Design review of the part built by this model. Coordinates are the model's own, in mm. A direction names the side the tool comes from. Round coordinates to 2 decimals unless told otherwise and drop trailing zeros. Loops run counter-clockwise (first coordinate to the right, second up) from the corner with the lowest first, then second, coordinate; pieces in that order, holes last. Notation, with made-up numbers: (83.5, 47.5) - (96.5, 47.5) arc R32 cw to (96.5, 86.5) - close; hole circle Ø5 at (33.5, 43). An arc over 180 degrees is marked (long way). Use one line per item in the form item = value. Start each with the question number.
(1) We need section B-B, the plane x = 23. Write out the cut boundary in (y, z).
(2) We need section D-D, the plane z = -26. Write out the cut boundary in (x, y).
(3) We need section C-C, the plane y = 10.5. Write out the cut boundary in (x, z), then the cut area to 3 significant figures.
(4) The part is to be moulded in two halves that separate along X. For faces 5 (the cylindrical face through (5.28, 5.92, 15.98)), 6 (the flat face through (45.311, 7, -40)), 7 (the flat face through (19, 2, -60.058)), say which applies: released by +X, released by -X, zero draft, split by the parting line, or undercut.
(5) Wall thickness on probe 1 along Z at (x, y) = (27.5, 1.75); probe 2 along X at (y, z) = (9.25, 15); probe 3 along X at (y, z) = (2, -98): over which ranges is each line inside the solid? List them lowest first. Write a range as [from, to].
(6) For pin 1 (3 mm diameter, centred on x = 7, z = 0, fed in from +Y); pin 2 (1 mm diameter, centred on x = 9.5, y = 13, fed in from +Z), all flat-tipped, find the tip position at first contact; note any pin that passes through.
(7) Machinability: for faces 1 (the flat face through (19, 12, 4)), 2 (the flat face through (19, 4, -41)), 3 (the flat face through (18, 14, -41)), 4 (the flat face through (19, 12, -85)), which of the approach directions +Z, -Z, +X, -X, +Y, -Y give a long, thin tool a straight path to every point of the face, cutting with its end or side? Answer none if there is none.
(8) We need section A-A, the plane y = 1.5. Write out the cut boundary in (x, z), then the cut area to 3 significant figures.
Autodesk Inventor part; units mm, degrees
ref_plane "YZ Plane" through (0, 0, 0) normal (1, 0, 0) x (0, 1, 0)
ref_plane "XZ Plane" through (0, 0, 0) normal (0, 1, 0) x (-1, 0, 0)
ref_plane "XY Plane" through (0, 0, 0) normal (0, 0, 1) x (1, 0, 0)
sketch "Sketch1" plane through (0, 0, 0) normal (0, 1, 0) x (-1, 0, 0)
  line L0 (3.6894, 22.9423) -> (-40.3106, 22.9423)
  line L1 (-45.3106, 17.9423) -> (-45.3106, -100.0577)
  line L2 (-40.3106, -105.0577) -> (3.6894, -105.0577)
  line L3 (8.6894, -100.0577) -> (8.6894, 17.9423)
  arc A0 (8.6894, 17.9423) -> (3.6894, 22.9423) centre (3.6894, 17.9423) ccw
  arc A1 (3.6894, -105.0577) -> (8.6894, -100.0577) centre (3.6894, -100.0577) ccw
  arc A2 (-40.3106, 22.9423) -> (-45.3106, 17.9423) centre (-40.3106, 17.9423) ccw
  arc A3 (-45.3106, -100.0577) -> (-40.3106, -105.0577) centre (-40.3106, -100.0577) ccw
  circle A4 centre (-1.3106, 12.9423) radius 5
  circle A5 centre (-1.3106, -95.0577) radius 5
  circle A6 centre (-35.3106, 12.9423) radius 5
  circle A7 centre (-35.3106, -95.0577) radius 5
  point P0 (0, 0)
  point P1 (-45.3106, -105.0577)
  point P2 (-45.3106, 22.9423)
  point P3 (8.6894, -105.0577)
  dimension "d0" = 54
  dimension "d1" = 128
  dimension "d2" = 5
  dimension "d3" = 5
  dimension "d4" = 5
  dimension "d5" = 5
  dimension "d6" = 10
  dimension "d7" = 10
  dimension "d8" = 10
  dimension "d9" = 10
  dimension "d10" = 10
  dimension "d11" = 10
  dimension "d12" = 10
  dimension "d13" = 10
  dimension "d14" = 10
  dimension "d15" = 10
  dimension "d16" = 10
  dimension "d17" = 10
extrude "Extrusion1" add sketch "Sketch1" along normal blind 12
sketch "Sketch2" plane through (0, 12, 0) normal (0, 1, 0) x (1, 0, 0)
  arc A0 (-8.6894, -17.9423) -> (-3.6894, -22.9423) centre (-3.6894, -17.9423) ccw
  line L0 (40.3106, 105.0577) -> (-3.6894, 105.0577)
  line L1 (-8.6894, 100.0577) -> (-8.6894, -17.9423)
  line L2 (-8.6894, 41.0577) -> (-8.6894, 16.0577)
  line L3 (-8.6894, 41.0577) -> (-8.6894, 66.0577)
  line L4 (-8.6894, 16.0577) -> (45.3106, 16.0577)
  line L5 (45.3106, -17.9423) -> (45.3106, 100.0577)
  line L6 (-8.6894, 66.0577) -> (45.3106, 66.0577)
  line L7 (45.3106, 66.0577) -> (45.3106, 16.0577)
  point P0 (0, 0)
  dimension "d21" = 25
  dimension "d22" = 25
extrude "Extrusion2" add sketch "Sketch2" along normal blind 2
sketch "Sketch3" plane through (45.3106, 0, 17.9423) normal (1, 0, 0) x (0, 0, -1)
  line L0 (34, 14) -> (59, 14)
  line L1 (118, 0) -> (0, 0)
  line L2 (59, 0) -> (40, 0)
  line L3 (59, 0) -> (78, 0)
  line L4 (40, 0) -> (40, 4)
  line L5 (78, 0) -> (78, 4)
  line L6 (78, 4) -> (40, 4)
  point P0 (17.9423, 0)
  dimension "d26" = 19
  dimension "d27" = 19
  dimension "d28" = 4
  dimension "d29" = 4
extrude "Extrusion3" cut sketch "Sketch3" against normal blind 54
properties part number "ttab"
Data:
q1.outline = (0, -105.06) - (12, -105.06) - (12, -66.06) - (14, -66.06) - (14, -16.06) - (12, -16.06) - (12, 22.94) - (0, 22.94) - (0, -22.06) - (4, -22.06) - (4, -60.06) - (0, -60.06) - close
q2.outline = (-8.69, 4) - (45.31, 4) - (45.31, 14) - (-8.69, 14) - close
q3.outline = (-8.69, -100.06) arc R5 ccw to (-3.69, -105.06) - (40.31, -105.06) arc R5 ccw to (45.31, -100.06) - (45.31, 17.94) arc R5 ccw to (40.31, 22.94) - (-3.69, 22.94) arc R5 ccw to (-8.69, 17.94) - close; hole circle Ø10 at (1.31, -95.06); hole circle Ø10 at (1.31, 12.94); hole circle Ø10 at (35.31, -95.06); hole circle Ø10 at (35.31, 12.94)
q3.area = 6,580 mm^2
q4.face_5 = undercut
q4.face_6 = released by +X
q4.face_7 = zero draft
q5.probe_1 = [-105.06, -60.06], [-22.06, 22.94]
q5.probe_2 = [-8.69, -3.25], [5.87, 30.75], [39.87, 45.31]
q5.probe_3 = [-8.69, -2.73], [5.35, 31.27], [39.35, 45.31]
q6.pin_1 = 12
q6.pin_2 = -16.06
q7.face_1 = +Z, +X, -X, +Y
q7.face_2 = +X, -X, -Y
q7.face_3 = +Z, -Z, +X, -X, +Y
q7.face_4 = -Z, +X, -X, +Y
q8.outline = (-8.69, -100.06) arc R5 ccw to (-3.69, -105.06) - (40.31, -105.06) arc R5 ccw to (45.31, -100.06) - (45.31, -60.06) - (-8.69, -60.06) - close; (-8.69, -22.06) - (45.31, -22.06) - (45.31, 17.94) arc R5 ccw to (40.31, 22.94) - (-3.69, 22.94) arc R5 ccw to (-8.69, 17.94) - close; hole circle Ø10 at (1.31, -95.06); hole circle Ø10 at (1.31, 12.94); hole circle Ø10 at (35.31, -95.06); hole circle Ø10 at (35.31, 12.94)
q8.area = 4,520 mm^2
